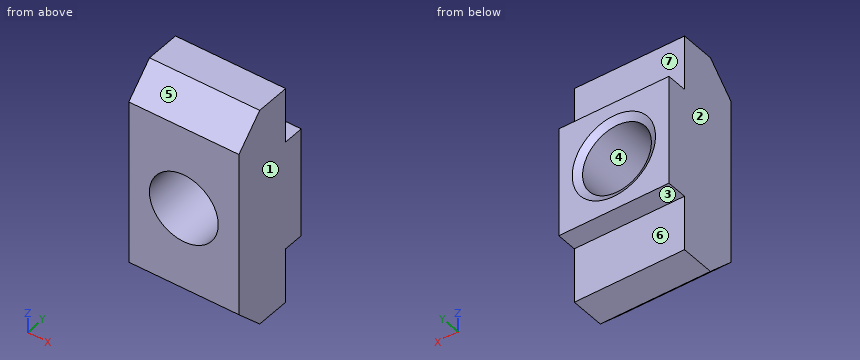
from build123d import *

# Parameters (mm, degrees)
SCHIZZO1_W                      = 8
SCHIZZO1_H                      = 6
ESTRUSIONE_ESTRUSIONE1_DEPTH    = 16
FORO_FILETTATO_M6_1_D           = 5
FORO_FILETTATO_M6_1_CSINK_D     = 6.05
FORO_FILETTATO_M6_1_CSINK_ANGLE = 120
SCHIZZO4_W                      = 4
SCHIZZO4_H                      = 1.5
TAGLIO_ESTRUSIONE1_DEPTH        = 10


with BuildPart() as part:
    # Schizzo1 → Estrusione-Estrusione1 (new body)
    with BuildSketch(Plane.XY):
        with Locations((0, 3)):
            Rectangle(SCHIZZO1_W, SCHIZZO1_H)
    extrude(amount=ESTRUSIONE_ESTRUSIONE1_DEPTH)

    # Foro filettato M6-1 (through all)
    with Locations(Plane(origin=(0, 6, 0), x_dir=(1, 0, 0), z_dir=(0, 1, 0))):
        with Locations((0, -8)):
            CounterSinkHole(FORO_FILETTATO_M6_1_D / 2, FORO_FILETTATO_M6_1_CSINK_D / 2, counter_sink_angle=FORO_FILETTATO_M6_1_CSINK_ANGLE)

    # Schizzo4 → Taglio-Estrusione1 (cut)
    with BuildSketch(Plane.ZY.offset(4)):
        Polygon((0, 0), (0, 2), (2, 0), align=None)
        Polygon((16, 0), (16, 2), (14, 0), align=None)
        with Locations((14, 5.25)):
            Rectangle(SCHIZZO4_W, SCHIZZO4_H)
        with Locations((2, 5.25)):
            Rectangle(SCHIZZO4_W, SCHIZZO4_H)
    extrude(amount=-TAGLIO_ESTRUSIONE1_DEPTH, mode=Mode.SUBTRACT)


solid = part.part
The listing builds one solid part. Answer for the finished solid, in the listing's coordinates (mm). Face numbers are marked on the shaded views. A direction names the side the tool comes from. Coordinates: 2 decimals unless noted, no trailing zeros. Loops run counter-clockwise (first coordinate to the right, second up) from the corner with the lowest first, then second, coordinate; pieces in that order, holes last.
1) Find the intervals of material crossed by L1, parallel to Z at x = 0, y = 2.7; L2, parallel to X at y = 4.25, z = 8; L3, parallel to Z at x = 0.5, y = 3.7, in increasing order.
2) Flat-ended cylindrical pins translate along their axes: pin 1 Ø2 at (x, z) = (0.5, 7) entering from -Y; pin 2 Ø1 at (x, y) = (-2, 5.5) entering from -Z; pin 3 Ø1.2 at (x, z) = (1, 14.5) entering from +Y. Find the tip coordinate at first contact, or state that the pin passes through.
3) Find section B-B on x = 0. Write down the section's boundary in (y, z) (3 decimals), then the cut area to 3 significant figures.
4) Find section C-C on y = 5.2. Write down the section's boundary in (x, z).
5) Find section D-D on x = 3.5. Write down the section's boundary in (y, z), then the cut area to 3 significant figures.
6) A tool of negligible diameter and unlimited length cuts with its end or side. For the marked faces 5, 6 and 7, from which of +Z, -Z, +X, -X, +Y, -Y can it reach the whole face along a straight path? Write none if from no direction.
7) Find section A-A on z = 8. Write down the section's boundary in (x, y) (3 decimals), then the cut area to 3 significant figures.
8) Determine the mould class of the marked faces 1, 2, 3 and 4 for opening direction X: pulls with the +X half, pulls with the -X half, needs draft (parallel to the pull), parting line crosses it, or undercut.
Values:
1. L1: z = 0 to 5.5, 10.5 to 16
1. L2: x = -4 to -2.5, 2.5 to 4
1. L3: z = 0 to 5.55, 10.45 to 16
2. pin 1: passes through
2. pin 2: stops at z = 4
2. pin 3: stops at y = 4.5
3. outline: (0, 2) - (2, 0) - (4.5, 0) - (4.5, 4) - (6, 4) - (6, 4.975) - (5.697, 5.5) - (0, 5.5) - close; (0, 10.5) - (5.697, 10.5) - (6, 11.025) - (6, 12) - (4.5, 12) - (4.5, 16) - (2, 16) - (0, 14) - close
3. area: 49.8 mm2
4. outline: (-4, 4) - (4, 4) - (4, 12) - (-4, 12) - close; hole circle Ø5 at (0, 8)
5. outline: (0, 2) - (2, 0) - (4.5, 0) - (4.5, 4) - (6, 4) - (6, 12) - (4.5, 12) - (4.5, 16) - (2, 16) - (0, 14) - close
5. area: 80.0 mm2
6. face 5: +Z, +X, -X, -Y
6. face 6: -Z, +X, -X, +Y
6. face 7: +Z, +X, -X, +Y
7. outline: (-4, 0) - (-2.5, 0) - (-2.5, 5.697) - (-3.025, 6) - (-4, 6) - close; (2.5, 0) - (4, 0) - (4, 6) - (3.025, 6) - (2.5, 5.697) - close
7. area: 17.8 mm2
8. face 1: pulls with the +X half
8. face 2: pulls with the -X half
8. face 3: needs draft
8. face 4: undercut
